Can you work these out from the model? Positions are in its coordinate system, mm. A direction names the side the tool comes from. Coordinates: 2 decimals unless noted, no trailing zeros. Order: outer loops, then holes, each group sorted by start corner. A loop starts at its lowest first (then second) coordinate and runs counter-clockwise, first axis right, second up. Notation, with made-up numbers: (41.5, 74.25) -> (55.5, 74.25) arc R24 ccw to (55.5, 87.25) -> close; hole circle Ø1 at (63.25, -26.5). An arc over 180 degrees is marked (long way). Answer in a Markdown table with one row per item. Add a question column.
1. Imagine slicing it at B-B on x = -18.5. Write out the boundary of the cut face in (y, z), plus the area to 3 significant figures.
2. Imagine slicing it at A-A on z = 29.5. Write out the boundary of the cut face in (x, y), plus the area to 3 significant figures.
3. If I drill on line 1 along Z through (x, y) = (0, -1.1); line 2 along Y through (x, z) = (1.5, 50.5), over which ranges is the centre line in solid material (lowest first)? Write a range as [from, to].
4. On a 3-axis mill with a long thin cutter (end or side, diameter ignored), from which of +Z, -Z, +X, -X, +Y, -Y can I reach the whole of each face in a straight line? I mean faces 1 (the face through (0, -3, 4)), 2 (the face through (29.305, 0.233, -16.524)). Say none if no direction works.
5. Will this pin go through, and if not, where does the flat tip stop? pin 1 (6.5 mm diameter, centred on x = 0, z = 0, fed in from +Y).
from build123d import *

# Parameters (mm, degrees)
SKETCH1_R           = 5.75
BOSS_EXTRUDE1_DEPTH = 3
BOSS_EXTRUDE2_DEPTH = 0.15
CIRPATTERN1_COUNT   = 3
SKETCH4_R           = 2.5
CUT_EXTRUDE1_DEPTH  = 7
CHAMFER1_SIZE       = 1


with BuildPart() as part:
    # Sketch1 → Boss-Extrude1 (new body, symmetric)
    with BuildSketch(Plane(origin=(0, 0, 0), x_dir=(1, 0, 0), z_dir=(0, 1, 0))):
        Circle(SKETCH1_R)
    extrude(amount=BOSS_EXTRUDE1_DEPTH, both=True)

    # Sketch3 → Boss-Extrude2 (add, symmetric)
    with BuildSketch(Plane(origin=(0, 0, 0), x_dir=(0.974370065, -0.224951054, 0), z_dir=(-0.224951054, -0.974370065, 0))):
        with BuildLine():
            Line((-3.401230627, 3.94493197), (-5.967495519, 6.417230684))
            Line((-5.967495519, 6.417230684), (-5.967495519, 60.5))
            ThreePointArc((-5.967495519, 60.5), (-5.088815862, 62.621320344), (-2.967495519, 63.5))
            Line((-2.967495519, 63.5), (-2.64407202, 63.5))
            ThreePointArc((-2.64407202, 63.5), (0.188980824, 62.61992859), (2.024718143, 60.289524634))
            ThreePointArc((2.024718143, 60.289524634), (4.284220879, 47.869969205), (5.041015214, 35.26925605))
            Line((5.041015214, 35.26925605), (5.041015214, 1.396310084))
            add(Edge.make_bspline(
                [(-3.401230627, 3.94493197), (1.650654294, 7.536977948), (5.041015214, 1.396310084)],
                knots=[0, 0, 0, 1, 1, 1], degree=2))
        make_face()
    boss_extrude2 = extrude(amount=BOSS_EXTRUDE2_DEPTH, both=True)

    # CirPattern1: Boss-Extrude2 ×3 about axis
    cirpattern1_axis = Axis((0, 0, 0), (0, 1, 0))
    for i in range(1, CIRPATTERN1_COUNT):
        add(boss_extrude2.rotate(cirpattern1_axis, i * 360 / CIRPATTERN1_COUNT))

    # Sketch4 → Cut-Extrude1 (cut, through all)
    with BuildSketch(Plane.XZ.offset(3)):
        Circle(SKETCH4_R)
    extrude(amount=-CUT_EXTRUDE1_DEPTH, mode=Mode.SUBTRACT)

    # Chamfer1
    chamfer1_edges = [part.edges().sort_by_distance(p)[0] for p in [
        (-2.5, 3, 0),
        (-2.5, -3, 0),
    ]]
    chamfer(chamfer1_edges, length=CHAMFER1_SIZE)


solid = part.part
Answers follow:
| question | item | result |
|---|---|---|
| 1 | outline | (-1.28, -5.05) -> (1.2, -17.43) -> (1.49, -17.36) -> (-0.99, -4.97) -> close |
| 1 | area | 3.81 mm² |
| 2 | outline | (-5.85, 1.2) -> (4.88, -1.28) -> (4.95, -0.99) -> (-5.78, 1.49) -> close |
| 2 | area | 3.30 mm² |
| 3 | line 1 | z = [-5.75, -2.5], [2.5, 5.75] |
| 3 | line 2 | y = [-0.5, -0.19] |
| 4 | face 1 | +Z, -Z, +X, -X, -Y |
| 4 | face 2 | -Z, +Y |
| 5 | pin 1 | stops at y = 2.75 |
